Could you check a few things on this model? Use its own coordinates, in mm. Face numbers are marked on the shaded views. A direction names the side the tool comes from. Round coordinates to 2 decimals unless told otherwise and drop trailing zeros. Loops run counter-clockwise (first coordinate to the right, second up) from the corner with the lowest first, then second, coordinate; pieces in that order, holes last. Notation, with made-up numbers: M 87.5,44.5 L 133.5,44.5 A4 cw 133.5,51.5 Z; hole C 65.5,88 d4. An arc over 180 degrees is marked long. Answer in a Markdown table with one row per item.
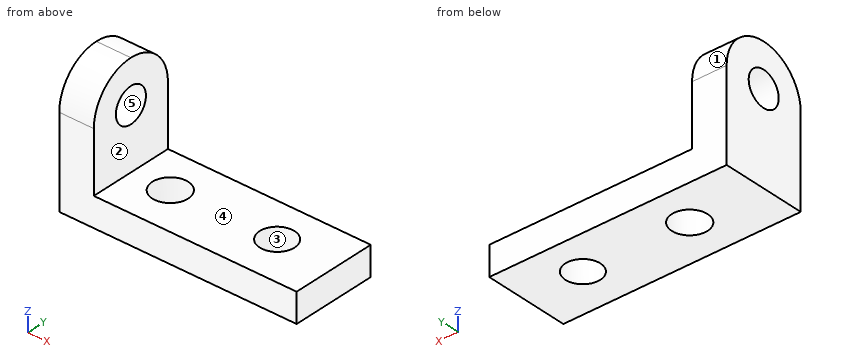
```python
from build123d import *

# Parameters (mm, degrees)
F1_DEPTH = 50
F2_R     = 24.99999
F3_R     = 10.4273095681
F3_R_2   = 10.1761827098
F4_DEPTH = 25
F5_R     = 10.1221707253
F6_DEPTH = 25


# Not quite as in the source:
# - a fillet or chamfer is up to 0.001 mm smaller than in the source, because OpenCascade refuses the exact size


with BuildPart() as f1:
    # F0 (on Front) → F1 (new body)
    with BuildSketch(Plane.XZ):
        Polygon((-87.5170975924, 9.8484745249), (-87.5170975924, -67.5976250101), (50.8091747761, -67.5976250101), (50.8091747761, -50.5853332579), (-67.3725008965, -50.5853332579), (-67.3725008965, 9.8484745249), align=None)
    extrude(amount=F1_DEPTH)

    # F2 (radius 25 in the source; OpenCascade refuses exactly that, so slightly less here)
    f2_edges = [f1.edges().sort_by_distance(p)[0] for p in [
        (-77.444799, -50, 9.848475),
        (-77.444799, 0, 9.848475),
    ]]
    fillet(f2_edges, radius=F2_R)

    # F3 (on face) → F4 (cut)
    with BuildSketch(Plane.XY.offset(-50.5853332579)):
        with Locations((-44.8602624238, -24.4600903243)):
            Circle(F3_R)
        with Locations((16.6889782995, -23.6502327025)):
            Circle(F3_R_2)
    extrude(amount=-F4_DEPTH, mode=Mode.SUBTRACT)

    # F5 (on face) → F6 (cut)
    with BuildSketch(Plane.YZ.offset(-67.3725008965)):
        with Locations((-25, -15.1515254751)):
            Circle(F5_R)
    extrude(amount=-F6_DEPTH, mode=Mode.SUBTRACT)


solid = f1.part
```
1) I want a section at B-B, the plane x = -48.5. Please give me the cut outline in (y, z), plus the area to 3 significant figures.
Computed:
| item | result |
|---|---|
| outline | M -50,-67.6 L -34.23,-67.6 L -34.23,-50.59 L -50,-50.59 Z; M -14.69,-67.6 L 0,-67.6 L 0,-50.59 L -14.69,-50.59 Z |
| area | 518 mm² |
2) I want a section at A-A, the plane y = -32. Please give me the cut outline in (x, z), plus the area to 3 significant figures.
Computed:
| item | result |
|---|---|
| outline | M -87.52,-67.6 L -52.06,-67.6 L -52.06,-50.59 L -67.37,-50.59 L -67.37,-22.46 L -87.52,-22.46 Z; M -87.52,-7.84 L -67.37,-7.84 L -67.37,8.85 L -87.52,8.85 Z; M -37.66,-67.6 L 10.87,-67.6 L 10.87,-50.59 L -37.66,-50.59 Z; M 22.51,-67.6 L 50.81,-67.6 L 50.81,-50.59 L 22.51,-50.59 Z |
| area | 2,810 mm² |
3) Which directions (+Z, -Z, +X, -X, +Y, -Y) give clear straight access to the entire face, cutting with the end or side of a thin tool? Please do the marked faces 1 and 2.
Computed:
| item | result |
|---|---|
| face 1 | +Z, +X, -X, +Y |
| face 2 | +Z, +X, +Y, -Y |
4) I want a section at D-D, the plane z = -27.5. Please give me the cut outline in (x, y).
Computed:
| item | result |
|---|---|
| outline | M -87.52,-50 L -67.37,-50 L -67.37,0 L -87.52,0 Z |
5) I want a section at C-C, the plane x = 17. Please give me the cut outline in (y, z), plus the area to 3 significant figures.
Computed:
| item | result |
|---|---|
| outline | M -50,-67.6 L -33.82,-67.6 L -33.82,-50.59 L -50,-50.59 Z; M -13.48,-67.6 L 0,-67.6 L 0,-50.59 L -13.48,-50.59 Z |
| area | 505 mm² |
6) Will these pins go through, and if not, where does the flat tip stop? P1, Ø23.5, axis at x = 16.69, y = -23.65, coming from the +Z side; P2, Ø6, axis at y = -6, z = -6.5, coming from the +X side; P3, Ø1.5, axis at x = 32.5, z = -48.5, coming from the +Y side.
Computed:
| item | result |
|---|---|
| P1 | stops at z = -50.59 |
| P2 | stops at x = -67.37 |
| P3 | passes through |
7) I need wall thicknesses on line 1 (Z direction, x = -83, y = -25); line 2 (Z direction, x = -57.5, y = -44.5); line 3 (X direction, y = -35, z = -47.5). Which ranges of each line are inside material? Lowest first, please.
Computed:
| item | result |
|---|---|
| line 1 | z = -67.6 to -25.27, -5.03 to 9.85 |
| line 2 | z = -67.6 to -50.59 |
| line 3 | x = -87.52 to -67.37 |
8) If we mould it in two halves opening along Z, with no side actions, what happens to the marked faces 3, 4 and 5? For each: released by +Z, released by -Z, zero draft, split by the parting line, or undercut.
Computed:
| item | result |
|---|---|
| face 3 | zero draft |
| face 4 | released by +Z |
| face 5 | undercut |
